from build123d import *

# Parameters (mm, degrees)
F0_W      = 150
F0_H      = 200
F0_R      = 12.5
F1_DEPTH  = 25
F3_DEPTH  = 100
F4_W      = 5
F4_H      = 100
F5_DEPTH  = 100
F7_DEPTH  = 25
F8_W      = 5
F8_H      = 100
F9_DEPTH  = 100
F11_DEPTH = 25


with BuildPart() as f1:
    # F0 (on Front) → F1 (new body)
    with BuildSketch(Plane.XZ):
        with Locations((75, -100)):
            Rectangle(F0_W, F0_H)
        with Locations((25, -175)):
            Circle(F0_R, mode=Mode.SUBTRACT)
        with Locations((125, -175)):
            Circle(F0_R, mode=Mode.SUBTRACT)
        with Locations((75, -25)):
            Circle(F0_R, mode=Mode.SUBTRACT)
    extrude(amount=F1_DEPTH)

    # F2 (on face) → F3 (join)
    with BuildSketch(Plane.XZ.offset(25)):
        with BuildLine():
            Line((42.5, -137.5), (37.5, -137.5))
            ThreePointArc((37.5, -137.5), (75, -175), (112.5, -137.5))
            Line((112.5, -137.5), (107.5, -137.5))
            ThreePointArc((107.5, -137.5), (75, -170), (42.5, -137.5))
        make_face()
    extrude(amount=F3_DEPTH)

    # F4 (on face) → F5 (join)
    with BuildSketch(Plane.XY.offset(-137.5)):
        with Locations((110, -75)):
            Rectangle(F4_W, F4_H)
    extrude(amount=F5_DEPTH)

    # F6 (on face) → F7 (cut)
    with BuildSketch(Plane.YZ.offset(112.5)):
        Polygon((-125, -37.5), (-125, -137.5), (-25, -37.5), align=None)
    extrude(amount=-F7_DEPTH, mode=Mode.SUBTRACT)

    # F8 (on face) → F9 (join)
    with BuildSketch(Plane.XY.offset(-137.5)):
        with Locations((40, -75)):
            Rectangle(F8_W, F8_H)
    extrude(amount=F9_DEPTH)

    # F10 (on face) → F11 (cut)
    with BuildSketch(Plane.YZ.offset(42.5)):
        Polygon((-125, -37.5), (-125, -137.5), (-25, -37.5), align=None)
    extrude(amount=-F11_DEPTH, mode=Mode.SUBTRACT)


solid = f1.part
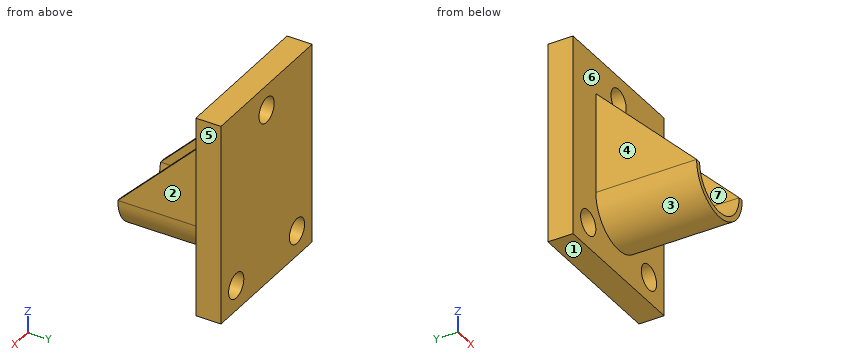
For this review, take the finished solid that the model builds, in its own axes (mm). Face numbers are marked on the shaded views. A direction names the side the tool comes from. Round coordinates to 2 decimals unless told otherwise and drop trailing zeros. Write each loop counter-clockwise with the first axis right and the second up, starting at its lowest first coordinate (ties: lowest second). Pieces come first, ordered by that corner, then holes. Notation, with made-up numbers: (74.5, -5.5) - (80.5, -5.5) arc R26 ccw to (80.5, 18.5) - close; hole circle Ø5 at (8, 13). An arc over 180 degrees is marked (long way). Use a Markdown table: item, result.
Q1. Clearance check with flat-ended pins moving along their axes: pin 1 (8 mm diameter, centred on x = 98, y = -63, fed in from -Z); pin 2 (10 mm diameter, centred on y = -71.5, z = -129, fed in from -X); pin 3 (1.5 mm diameter, centred on y = -55, z = -141, fed in from -X). State where each tip first meets the part, or that it passes through.
Derived:
| item | result |
|---|---|
| pin 1 | stops at z = -169.83 |
| pin 2 | stops at x = 37.5 |
| pin 3 | stops at x = 37.6 |
Q2. We need section D-D (z = -85). Give the boundary of the cut face in (x, y), plus the area to 4 significant figures.
Derived:
| item | result |
|---|---|
| outline | (0, -25) - (37.5, -25) - (37.5, -72.5) - (42.5, -72.5) - (42.5, -25) - (107.5, -25) - (107.5, -72.5) - (112.5, -72.5) - (112.5, -25) - (150, -25) - (150, 0) - (0, 0) - close |
| area | 4,225 mm2 |
Q3. Wall thickness on line 1 along Z through (x, y) = (125, -11); line 2 along Z through (x, y) = (75, -10); line 3 along Y through (x, z) = (79.5, -89): over which ranges is each line inside the solid? List them lowest first.
Derived:
| item | result |
|---|---|
| line 1 | z = -200 to -187.5, -162.5 to 0 |
| line 2 | z = -200 to -37.5, -12.5 to 0 |
| line 3 | y = -25 to 0 |
Q4. We need section C-C (y = -13). Give the boundary of the cut face in (x, z), plus the area to 3 significant figures.
Derived:
| item | result |
|---|---|
| outline | (0, -200) - (150, -200) - (150, 0) - (0, 0) - close; hole circle Ø25 at (25, -175); hole circle Ø25 at (75, -25); hole circle Ø25 at (125, -175) |
| area | 28,500 mm2 |
Q5. Machinability: for the marked faces 1, 2 and 3, which of the approach directions +Z, -Z, +X, -X, +Y, -Y give a long, thin tool a straight path to every point of the face, cutting with its end or side? Answer none if there is none.
Derived:
| item | result |
|---|---|
| face 1 | -Z, +X, -X, +Y, -Y |
| face 2 | +Z, -Z, +X, -Y |
| face 3 | -Z, -Y |
Q6. We need section B-B (z = -25). Give the boundary of the cut face in (x, y), plus the area to 4 significant figures.
Derived:
| item | result |
|---|---|
| outline | (0, -25) - (62.5, -25) - (62.5, 0) - (0, 0) - close; (87.5, -25) - (150, -25) - (150, 0) - (87.5, 0) - close |
| area | 3,125 mm2 |
Q7. The part is to be moulded in two halves that separate along X. For the marked faces 4, 5, 6 and 7, say which applies: pulls with the +X half, pulls with the -X half, needs draft (parallel to the pull), parting line crosses it, or undercut.
Derived:
| item | result |
|---|---|
| face 4 | pulls with the -X half |
| face 5 | pulls with the +X half |
| face 6 | undercut |
| face 7 | undercut |
Q8. We need section A-A (x = 75). Give the boundary of the cut face in (y, z).
Derived:
| item | result |
|---|---|
| outline | (-125, -175) - (-25, -175) - (-25, -200) - (0, -200) - (0, -37.5) - (-25, -37.5) - (-25, -170) - (-125, -170) - close; (-25, -12.5) - (0, -12.5) - (0, 0) - (-25, 0) - close |
